Study the drawing (mm; zero at the part's minimum x, y, z) and answer. Give positions to 0.01 mm unless a question says otherwise; leave off trailing zeros. Loops run counter-clockwise (first coordinate to the right, second up) from the corner with the lowest first, then second, coordinate; pieces in that order, holes last. Notation, with made-up numbers: (-23.5, -12) - (34.5, -12) arc R15 cw to (34.5, -3) - close; hole circle Ø6 at (-8.75, 66.5). An arc over 180 degrees is marked (long way). One line per item, written item: value. Start each with the question number.
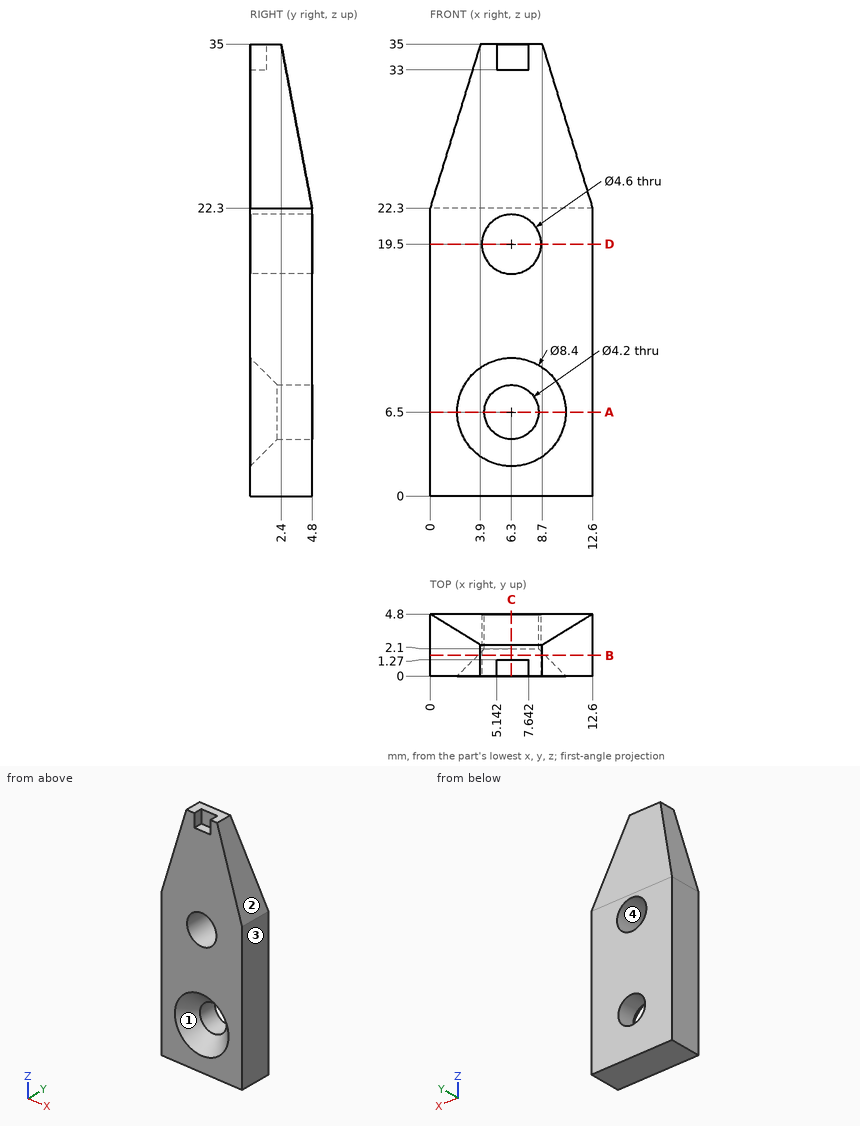
1. A cutting plane is placed at D-D (z = 19.5). Determine the outline of the cut face in (x, y), plus the area to 3 significant figures.
2. Flat-ended cylindrical pins translate along their axes: pin 1 (1.4 mm diameter, centred on x = 6, y = 0.5, fed in from +Z); pin 2 (5.5 mm diameter, centred on x = 6.3, z = 6.5, fed in from -Y); pin 3 (0.6 mm diameter, centred on y = 0.5, z = 34, fed in from +X); pin 4 (4 mm diameter, centred on x = 6.3, z = 19.5, fed in from -Y). Find the tip coordinate at first contact, or state that the pin passes through.
3. A cutting plane is placed at C-C (x = 6.3). Give the number of separate pieces and of enclosed holes in the cut face, plus the area to 3 significant figures.
4. Find the intervals of material crossed by L1, parallel to X at y = 2.95, z = 6.5; L2, parallel to Z at x = 6.5, y = 0.3 (1 decimal); L3, parallel to Y at x = 2.5, z = 25.5 (1 decimal), in increasing order. Write a range as [from, to].
5. A cutting plane is placed at B-B (y = 1.6). Determine the outline of the cut face in (x, z).
6. A cutting plane is placed at A-A (z = 6.5). Determine the outline of the cut face in (x, y), plus the area to 3 significant figures.
7. Determine the mould class of the marked faces 1, 2, 3 and 4 for opening direction Z: released by +Z, released by -Z, zero draft, split by the parting line, or undercut.
Results below:
1. outline: (0, 0) - (4, 0) - (4, 4.8) - (0, 4.8) - close; (8.6, 0) - (12.6, 0) - (12.6, 4.8) - (8.6, 4.8) - close
1. area: 38.4 mm^2
2. pin 1: stops at z = 33
2. pin 2: stops at y = 1.45
2. pin 3: stops at x = 9.1
2. pin 4: passes through
3. separate pieces: 3
3. enclosed holes: 0
3. area: 104 mm^2
4. L1: x = [0, 4.2], [8.4, 12.6]
4. L2: z = [0, 2.6], [10.4, 17.2], [21.8, 33]
4. L3: y = [0, 4.2]
5. outline: (0, 0) - (12.6, 0) - (12.6, 22.3) - (8.7, 35) - (3.9, 35) - (0, 22.3) - close; hole circle Ø5.2 at (6.3, 6.5); hole circle Ø4.6 at (6.3, 19.5)
6. outline: (0, 0) - (2.1, 0) - (4.2, 2.1) - (4.2, 4.8) - (0, 4.8) - close; (8.4, 2.1) - (10.5, 0) - (12.6, 0) - (12.6, 4.8) - (8.4, 4.8) - close
6. area: 35.9 mm^2
7. face 1: undercut
7. face 2: released by +Z
7. face 3: zero draft
7. face 4: undercut
